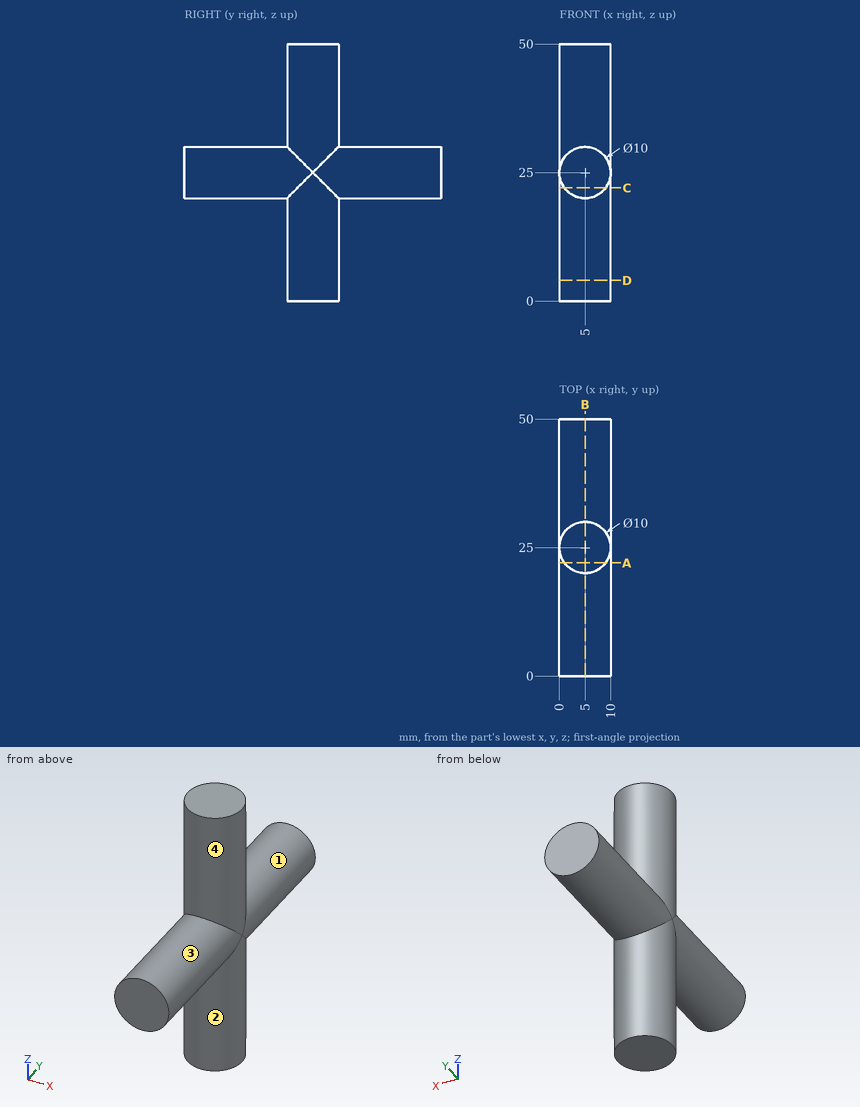
Can you work these out from the drawing? Everything is in mm from the part's minimum corner. A direction names the side the tool comes from. Round coordinates to 2 decimals unless told otherwise and drop trailing zeros. Write each loop counter-clockwise with the first axis right and the second up, starting at its lowest first coordinate (ties: lowest second). Pieces come first, ordered by that corner, then holes. Notation, with made-up numbers: (9.25, 29) - (53.25, 29) arc R8 ccw to (53.25, 41) - close; hole circle Ø9 at (39, 24.5). An arc over 180 degrees is marked (long way). Put each result on its own line as item: value. Start each with the question number.
(1) I want a section at B-B, the plane x = 5. Please give me the cut outline in (y, z).
(2) I want a section at A-A, the plane y = 22. Please give me the cut outline in (x, z), plus the area to 3 significant figures.
(3) I need wall thicknesses on probe 1 along Z at (x, y) = (5.25, 43); probe 2 along Y at (x, z) = (5, 41.5); probe 3 along Z at (x, y) = (1.25, 35.5). Which ranges of each line are inside material? Lowest first, please.
(4) For the marked faces 1, 2, 3 and 4, which set-ups out of +Z, -Z, +X, -X, +Y, -Y let a thin tool reach every point of the face, with its end or its side?
(5) Will these pins go through, and if not, where does the flat tip stop? pin 1 (4 mm diameter, centred on x = 4.5, y = 36.5, fed in from +Z); pin 2 (1 mm diameter, centred on y = 27, z = 39, fed in from +X); pin 3 (1.5 mm diameter, centred on x = 8.5, y = 37, fed in from +Z).
(6) I want a section at D-D, the plane z = 4. Please give me the cut outline in (x, y), plus the area to 3 significant figures.
Here are the results:
1. outline: (0, 20) - (20, 20) - (20, 0) - (30, 0) - (30, 20) - (50, 20) - (50, 30) - (30, 30) - (30, 50) - (20, 50) - (20, 30) - (0, 30) - close
2. outline: (1, 0) - (9, 0) - (9, 22) arc R5 ccw to (9, 28) - (9, 50) - (1, 50) - (1, 28) arc R5 ccw to (1, 22) - close
2. area: 408 mm^2
3. probe 1: z = 20.01 to 29.99
3. probe 2: y = 20 to 30
3. probe 3: z = 21.69 to 28.31
4. face 1: +Y
4. face 2: -Z
4. face 3: -Y
4. face 4: +Z
5. pin 1: stops at z = 30
5. pin 2: stops at x = 9.77
5. pin 3: stops at z = 29.18
6. outline: circle Ø10 at (5, 25)
6. area: 78.5 mm^2
